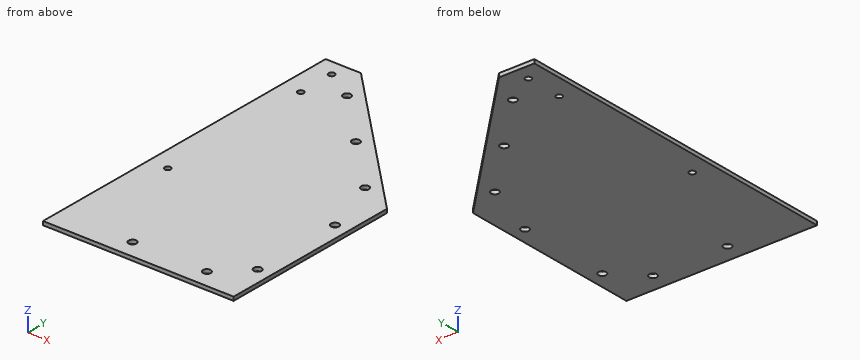
```python
from build123d import *

# Parameters (mm, degrees)
SKETCH_1_R          = 2.1
EXTRUDE_1_DEPTH     = 2
SKETCH_2_R          = 2.1
CUT_EXTRUDE_1_DEPTH = 10
M4X0_7_1_OUTLINE_W  = 19
M4X0_7_1_OUTLINE_H  = 182.73
M4X0_7_1_OUTLINE_R  = 1.65
M4X0_7_1_DEPTH      = 2


# Read off the part's stored shape, not the designer's step: M4x0.7 ねじ穴1
with BuildPart() as part:
    # ｽｹｯﾁ1 → ﾎﾞｽ - 押し出し1 (new body)
    with BuildSketch(Plane.XY):
        Polygon((0, 0), (0, 182.73), (83.56, 99.17), (83.56, 0), align=None)
        with Locations((8.132919651, 163.990478631)):
            Circle(SKETCH_1_R, mode=Mode.SUBTRACT)
        with Locations((36.417190898, 135.706207384)):
            Circle(SKETCH_1_R, mode=Mode.SUBTRACT)
        with Locations((64.91002614, 107.428490375)):
            Circle(SKETCH_1_R, mode=Mode.SUBTRACT)
        with Locations((76.06, 74.59)):
            Circle(SKETCH_1_R, mode=Mode.SUBTRACT)
        with Locations((76.06, 24.59)):
            Circle(SKETCH_1_R, mode=Mode.SUBTRACT)
    extrude(amount=EXTRUDE_1_DEPTH)

    # ｽｹｯﾁ2 → ｶｯﾄ - 押し出し1 (cut)
    with BuildSketch(Plane.XY.offset(2)):
        with Locations((21.12, 9.69)):
            Circle(SKETCH_2_R)
        with Locations((61.12, 9.69)):
            Circle(SKETCH_2_R)
    extrude(amount=-CUT_EXTRUDE_1_DEPTH, mode=Mode.SUBTRACT)

    # M4x0.7 ねじ穴1 outline → M4x0.7 ねじ穴1 (add)
    with BuildSketch(Plane.XY):
        with Locations((-9.5, 91.365)):
            Rectangle(M4X0_7_1_OUTLINE_W, M4X0_7_1_OUTLINE_H)
        with Locations((-8.59, 68.15)):
            Circle(M4X0_7_1_OUTLINE_R, mode=Mode.SUBTRACT)
        with Locations((-8.59, 154.15)):
            Circle(M4X0_7_1_OUTLINE_R, mode=Mode.SUBTRACT)
        with Locations((-8.59, 174.15)):
            Circle(M4X0_7_1_OUTLINE_R, mode=Mode.SUBTRACT)
    extrude(amount=M4X0_7_1_DEPTH)


solid = part.part
```
Source: CAD feature listing. Evaluate the final solid. Frame: model axes, mm. Give positions to 0.01 mm unless a question says otherwise; leave off trailing zeros. Loops run counter-clockwise (first coordinate to the right, second up) from the corner with the lowest first, then second, coordinate; pieces in that order, holes last. Notation, with made-up numbers: (41.25, 30) -> (66.25, 30) arc R35 ccw to (66.25, 64) -> close; hole circle Ø1 at (-0.75, 80). An arc over 180 degrees is marked (long way). Use a Markdown table: item, result. Add a question column.
(1) Section query A-A (y = 24.59). Output: boundary loops of the cut face in (x, z).
(2) Section query B-B (x = 76.06). Output: boundary loops of the cut face in (y, z).
(3) Section query D-D (z = 1.6). Count the separate pieces of the cut face and the enclosed holes in it, then the cut area to 3 significant figures.
(4) Ray query, line 1 (Y direction, x = -8.59, z = 1.25); line 2 (Y direction, x = 76, z = 1.7); line 3 (Y direction, x = 60, z = 1.7). Return the intervals inside material, ascending.
(5) Section query C-C (x = 21.12). Output: boundary loops of the cut face in (y, z).
(6) First-contact query: pin 1 Ø5 at (x, y) = (8.13, 163.99) entering from +Z. Flat tip, straight axial feed; report the tip coordinate or a pass-through.
Checked values:
| question | item | result |
|---|---|---|
| 1 | outline | (-19, 0) -> (73.96, 0) -> (73.96, 2) -> (-19, 2) -> close; (78.16, 0) -> (83.56, 0) -> (83.56, 2) -> (78.16, 2) -> close |
| 2 | outline | (0, 0) -> (22.49, 0) -> (22.49, 2) -> (0, 2) -> close; (26.69, 0) -> (72.49, 0) -> (72.49, 2) -> (26.69, 2) -> close; (76.69, 0) -> (106.67, 0) -> (106.67, 2) -> (76.69, 2) -> close |
| 3 | separate pieces | 1 |
| 3 | enclosed holes | 10 |
| 3 | area | 15,100 mm^2 |
| 4 | line 1 | 0 to 66.5, 69.8 to 152.5, 155.8 to 172.5, 175.8 to 182.73 |
| 4 | line 2 | 0 to 22.49, 26.69 to 72.49, 76.69 to 106.73 |
| 4 | line 3 | 0 to 7.91, 11.47 to 122.73 |
| 5 | outline | (0, 0) -> (7.59, 0) -> (7.59, 2) -> (0, 2) -> close; (11.79, 0) -> (161.61, 0) -> (161.61, 2) -> (11.79, 2) -> close |
| 6 | pin 1 | z = 2 |
